```python
from build123d import *

# Parameters (mm, degrees)
F0_W     = 838.2
F0_H     = 82.55
F1_DEPTH = 6.35
F3_DEPTH = 6.35
F5_DEPTH = 6.35


# Not quite as in the source:
# - a pattern or mirror of a feature is missing from the dataset's text; its kind, count and spacing are read off the source's solid


with BuildPart() as f1:
    # F0 (on Front) → F1 (new body)
    with BuildSketch(Plane.XZ):
        Rectangle(F0_W, F0_H)
    extrude(amount=F1_DEPTH)

    # F2 (on face) → F3 (cut, through all)
    with BuildSketch(Plane.XZ.offset(6.35)):
        with BuildLine():
            ThreePointArc((-267.208, 15.24), (-270.6768409794, 16.6768409794), (-269.24, 13.208))
            Line((-269.24, 13.208), (-269.24, 15.24))
            Line((-269.24, 15.24), (-267.208, 15.24))
        make_face()
        with BuildLine():
            Line((-269.24, 15.24), (-269.24, 13.208))
            ThreePointArc((-269.24, 13.208), (-267.8031590206, 13.8031590206), (-267.208, 15.24))
            Line((-267.208, 15.24), (-269.24, 15.24))
        make_face()
        with BuildLine():
            Line((-254, 0), (-268.2875, 0))
            ThreePointArc((-268.2875, 0), (-254, -14.2875), (-239.7125, 0))
            ThreePointArc((-239.7125, 0), (-243.8972118638, 10.1027881362), (-254, 14.2875))
            Line((-254, 14.2875), (-254, 0))
        make_face()
        with BuildLine():
            ThreePointArc((-254, 14.2875), (-264.1027881362, 10.1027881362), (-268.2875, 0))
            Line((-268.2875, 0), (-254, 0))
            Line((-254, 0), (-254, 14.2875))
        make_face()
        with BuildLine():
            Line((-269.24, -15.24), (-269.24, -13.208))
            ThreePointArc((-269.24, -13.208), (-270.6768409794, -16.6768409794), (-267.208, -15.24))
            Line((-267.208, -15.24), (-269.24, -15.24))
        make_face()
        with BuildLine():
            ThreePointArc((-267.208, -15.24), (-267.8031590206, -13.8031590206), (-269.24, -13.208))
            Line((-269.24, -13.208), (-269.24, -15.24))
            Line((-269.24, -15.24), (-267.208, -15.24))
        make_face()
        with BuildLine():
            Line((-238.76, -15.24), (-240.792, -15.24))
            ThreePointArc((-240.792, -15.24), (-238.76, -17.272), (-236.728, -15.24))
            ThreePointArc((-236.728, -15.24), (-237.3231590206, -13.8031590206), (-238.76, -13.208))
            Line((-238.76, -13.208), (-238.76, -15.24))
        make_face()
        with BuildLine():
            ThreePointArc((-238.76, -13.208), (-240.1968409794, -13.8031590206), (-240.792, -15.24))
            Line((-240.792, -15.24), (-238.76, -15.24))
            Line((-238.76, -15.24), (-238.76, -13.208))
        make_face()
        with BuildLine():
            ThreePointArc((-236.728, 15.24), (-240.1968409794, 16.6768409794), (-238.76, 13.208))
            ThreePointArc((-238.76, 13.208), (-237.3231590206, 13.8031590206), (-236.728, 15.24))
        make_face()
        with BuildLine():
            ThreePointArc((14.2875, 0), (10.1027881362, 10.1027881362), (0, 14.2875))
            ThreePointArc((0, 14.2875), (-10.1027881362, -10.1027881362), (14.2875, 0))
        make_face()
        with BuildLine():
            Line((15.24, -15.24), (13.208, -15.24))
            ThreePointArc((13.208, -15.24), (15.24, -17.272), (17.272, -15.24))
            ThreePointArc((17.272, -15.24), (16.6768409794, -13.8031590206), (15.24, -13.208))
            Line((15.24, -13.208), (15.24, -15.24))
        make_face()
        with BuildLine():
            ThreePointArc((15.24, -13.208), (13.8031590206, -13.8031590206), (13.208, -15.24))
            Line((13.208, -15.24), (15.24, -15.24))
            Line((15.24, -15.24), (15.24, -13.208))
        make_face()
        with BuildLine():
            ThreePointArc((17.272, 15.24), (13.8031590206, 16.6768409794), (15.24, 13.208))
            ThreePointArc((15.24, 13.208), (16.6768409794, 13.8031590206), (17.272, 15.24))
        make_face()
        with BuildLine():
            Line((-15.24, 15.24), (-13.208, 15.24))
            ThreePointArc((-13.208, 15.24), (-16.6768409794, 16.6768409794), (-15.24, 13.208))
            Line((-15.24, 13.208), (-15.24, 15.24))
        make_face()
        with BuildLine():
            ThreePointArc((-15.24, 13.208), (-13.8031590206, 13.8031590206), (-13.208, 15.24))
            Line((-13.208, 15.24), (-15.24, 15.24))
            Line((-15.24, 15.24), (-15.24, 13.208))
        make_face()
        with BuildLine():
            Line((-15.24, -15.24), (-15.24, -13.208))
            ThreePointArc((-15.24, -13.208), (-16.6768409794, -16.6768409794), (-13.208, -15.24))
            Line((-13.208, -15.24), (-15.24, -15.24))
        make_face()
        with BuildLine():
            ThreePointArc((-13.208, -15.24), (-13.8031590206, -13.8031590206), (-15.24, -13.208))
            Line((-15.24, -13.208), (-15.24, -15.24))
            Line((-15.24, -15.24), (-13.208, -15.24))
        make_face()
    f3 = extrude(amount=-F3_DEPTH, mode=Mode.SUBTRACT)

    # F3_copies: F3 across plane
    add(f3.mirror(Plane(origin=(0, 0, 0), x_dir=(0, 0, 1), z_dir=(1, 0, 0))), mode=Mode.SUBTRACT)

    # F4 (on face) → F5 (cut, through all)
    with BuildSketch(Plane.XZ.offset(6.35)):
        with BuildLine():
            ThreePointArc((-403.86, 26.035), (-404.6039487758, 27.8310512242), (-406.4, 28.575))
            Line((-406.4, 28.575), (-406.4, 23.495))
            ThreePointArc((-406.4, 23.495), (-404.6039487758, 24.2389487758), (-403.86, 26.035))
        make_face()
        with BuildLine():
            ThreePointArc((-403.86, -26.035), (-404.6039487758, -24.2389487758), (-406.4, -23.495))
            Line((-406.4, -23.495), (-406.4, -28.575))
            ThreePointArc((-406.4, -28.575), (-404.6039487758, -27.8310512242), (-403.86, -26.035))
        make_face()
        with BuildLine():
            Line((-406.4, -28.575), (-406.4, -23.495))
            ThreePointArc((-406.4, -23.495), (-408.94, -26.035), (-406.4, -28.575))
        make_face()
        with BuildLine():
            Line((-406.4, 23.495), (-406.4, 28.575))
            ThreePointArc((-406.4, 28.575), (-408.94, 26.035), (-406.4, 23.495))
        make_face()
        with BuildLine():
            ThreePointArc((-124.46, 26.035), (-125.2039487758, 27.8310512242), (-127, 28.575))
            Line((-127, 28.575), (-127, 23.495))
            ThreePointArc((-127, 23.495), (-125.2039487758, 24.2389487758), (-124.46, 26.035))
        make_face()
        with BuildLine():
            ThreePointArc((-124.46, -26.035), (-125.2039487758, -24.2389487758), (-127, -23.495))
            Line((-127, -23.495), (-127, -28.575))
            ThreePointArc((-127, -28.575), (-125.2039487758, -27.8310512242), (-124.46, -26.035))
        make_face()
        with BuildLine():
            Line((-127, -28.575), (-127, -23.495))
            ThreePointArc((-127, -23.495), (-129.54, -26.035), (-127, -28.575))
        make_face()
        with BuildLine():
            Line((-127, 23.495), (-127, 28.575))
            ThreePointArc((-127, 28.575), (-129.54, 26.035), (-127, 23.495))
        make_face()
    f5 = extrude(amount=-F5_DEPTH, mode=Mode.SUBTRACT)

    # F5_copies: F5 across plane
    add(f5.mirror(Plane(origin=(0, 0, 0), x_dir=(0, 0, 1), z_dir=(1, 0, 0))), mode=Mode.SUBTRACT)


solid = f1.part
```
Geometry: final body of the model. Coordinates: model frame, mm. Coordinates: 2 decimals unless noted, no trailing zeros. Order: outer loops, then holes, each group sorted by start corner. A loop starts at its lowest first (then second) coordinate and runs counter-clockwise, first axis right, second up. Notation, with made-up numbers: (-34, 44.5) -> (-14, 44.5) arc R28 cw to (-14, 76.5) -> close; hole circle Ø1 at (49.5, 59.25). An arc over 180 degrees is marked (long way). Answer in a Markdown table with one row per item.
Item 1: Draft query along X for faces 1 (the flat face through (-6, 0, -18)), 2 (the cylindrical face through (-14.166, -3.219, -1.86)). Return one class per face: released by +X, released by -X, zero draft, split by the parting line, or undercut.
Return value:
| item | result |
|---|---|
| face 1 | zero draft |
| face 2 | undercut |
Item 2: Section C-C on y = -4. State how many separate pieces and enclosed holes the cut face has, plus the area to 3 significant figures.
Return value:
| item | result |
|---|---|
| separate pieces | 1 |
| enclosed holes | 23 |
| area | 67,000 mm² |
Item 3: Section B-B on z = -5. Output: boundary loops of the cut face in (x, y), plus the area to 3 significant figures.
Return value:
| item | result |
|---|---|
| outline | (-419.1, -6.35) -> (-267.38, -6.35) -> (-267.38, 0) -> (-419.1, 0) -> close; (-240.62, -6.35) -> (-13.38, -6.35) -> (-13.38, 0) -> (-240.62, 0) -> close; (13.38, -6.35) -> (240.62, -6.35) -> (240.62, 0) -> (13.38, 0) -> close; (267.38, -6.35) -> (419.1, -6.35) -> (419.1, 0) -> (267.38, 0) -> close |
| area | 4,810 mm² |
Item 4: Ray query, L1, parallel to Z at x = 269.24, y = -2.25 (3 decimals); L2, parallel to X at y = -1, z = 26.5; L3, parallel to X at y = -5.25, z = 1.5. Return the intervals inside material, ascending.
Return value:
| item | result |
|---|---|
| L1 | z = -41.275 to -17.272, -13.208 to 13.208, 17.272 to 41.275 |
| L2 | x = -419.1 to -408.9, -403.9 to -129.5, -124.5 to 124.5, 129.5 to 403.9, 408.9 to 419.1 |
| L3 | x = -419.1 to -268.21, -239.79 to -14.21, 14.21 to 239.79, 268.21 to 419.1 |
